from build123d import *

# Parameters (mm, degrees)
SKETCH1_W                   = 76.2
SKETCH1_H                   = 38.1
SKETCH1_W_2                 = 69.85
SKETCH1_H_2                 = 31.75
BOSS_EXTRUDE1_DEPTH         = 311.15
F_1_4_20_TAPPED_HOLE1_D     = 5.1054
F_1_4_20_TAPPED_HOLE1_DEPTH = 3.175


with BuildPart() as part:
    # Sketch1 → Boss-Extrude1 (new body, symmetric)
    with BuildSketch(Plane(origin=(0, 0, 0), x_dir=(0, 0, -1), z_dir=(1, 0, 0))):
        with Locations((38.1, 19.05)):
            Rectangle(SKETCH1_W, SKETCH1_H)
        with Locations((38.1, 19.05)):
            Rectangle(SKETCH1_W_2, SKETCH1_H_2, mode=Mode.SUBTRACT)
    extrude(amount=BOSS_EXTRUDE1_DEPTH, both=True)

    # 1/4-20 Tapped Hole1
    with Locations(Plane(origin=(0, 0, -76.2), x_dir=(-1, 0, 0), z_dir=(0, 0, -1))):
        with Locations((260.35, 19.05), (-260.35, 19.05)):
            Hole(F_1_4_20_TAPPED_HOLE1_D / 2, depth=F_1_4_20_TAPPED_HOLE1_DEPTH)


solid = part.part
The listing builds one solid part. Answer for the finished solid, in the listing's coordinates (mm). A direction names the side the tool comes from. Round coordinates to 2 decimals unless told otherwise and drop trailing zeros. Order: outer loops, then holes, each group sorted by start corner. A loop starts at its lowest first (then second) coordinate and runs counter-clockwise, first axis right, second up. Notation, with made-up numbers: (71.5, 47) -> (81.5, 47) arc R12 ccw to (81.5, 55) -> close; hole circle Ø2 at (34, 63.25). An arc over 180 degrees is marked (long way). Put each result on its own line as item: value.
Q1. Consider line 1 along Z through (x, y) = (-150, 21) (3 decimals); line 2 along Y through (x, z) = (-134, -51) (3 decimals); line 3 along Y through (x, z) = (-260, -75). Determine where each line is inside the solid, lowest interval first.
Results list:
line 1: -76.2 to -73.025, -3.175 to 0
line 2: 0 to 3.175, 34.925 to 38.1
line 3: 0 to 16.52, 21.58 to 38.1
Q2. This flat-tipped pin is pushed along its axis until it touches: P1, Ø4, axis at x = -260.35, y = 19.05, coming from the -Z side (3 decimals). Where does it stop, or does it pass through?
Results list:
P1: z = -3.175
Q3. Section A-A, the plane z = -53 is taken. Write down the section's boundary in (x, y) (3 decimals), and give its area (3 significant figures).
Results list:
outline: (-311.15, 0) -> (311.15, 0) -> (311.15, 3.175) -> (-311.15, 3.175) -> close; (-311.15, 34.925) -> (311.15, 34.925) -> (311.15, 38.1) -> (-311.15, 38.1) -> close
area: 3,950 mm^2
Q4. Determine the mould class of faces 3 (the flat face through (4, 19, 0)), 4 (the flat face through (4, 34.925, -38)), 5 (the flat face through (4, 19, -76.2)), 6 (the flat face through (4, 0, -38)) for opening direction Z: pulls with the +Z half, pulls with the -Z half, needs draft (parallel to the pull), parting line crosses it, or undercut.
Results list:
face 3: pulls with the +Z half
face 4: undercut
face 5: pulls with the -Z half
face 6: needs draft
Q5. Section B-B, the plane x = -96.5 is taken. Write down the section's boundary in (y, z) (3 decimals), and give its area (3 significant figures).
Results list:
outline: (0, -76.2) -> (38.1, -76.2) -> (38.1, 0) -> (0, 0) -> close; hole (3.175, -73.025) -> (34.925, -73.025) -> (34.925, -3.175) -> (3.175, -3.175) -> close
area: 685 mm^2
Q6. Which of the six approach directions +Z, -Z, +X, -X, +Y, -Y give full straight-line access (tool end or side, diameter ignored) to faces 1 (the flat face through (4, 19, -3.175)), 2 (the flat face through (311.15, 2, -35))?
Results list:
face 1: +X, -X
face 2: +Z, -Z, +X, +Y, -Y
